The drawing under review shows one solid part. Ordinate dimensions are in mm from its lowest x, y, z. Round coordinates to 2 decimals unless told otherwise and drop trailing zeros. Order: outer loops, then holes, each group sorted by start corner. A loop starts at its lowest first (then second) coordinate and runs counter-clockwise, first axis right, second up. Notation, with made-up numbers: M 43.5,-36.5 L 82.5,-36.5 A13 ccw 82.5,-27.5 Z; hole C 20.5,23 d7. An arc over 180 degrees is marked long. Use a Markdown table: item, result.
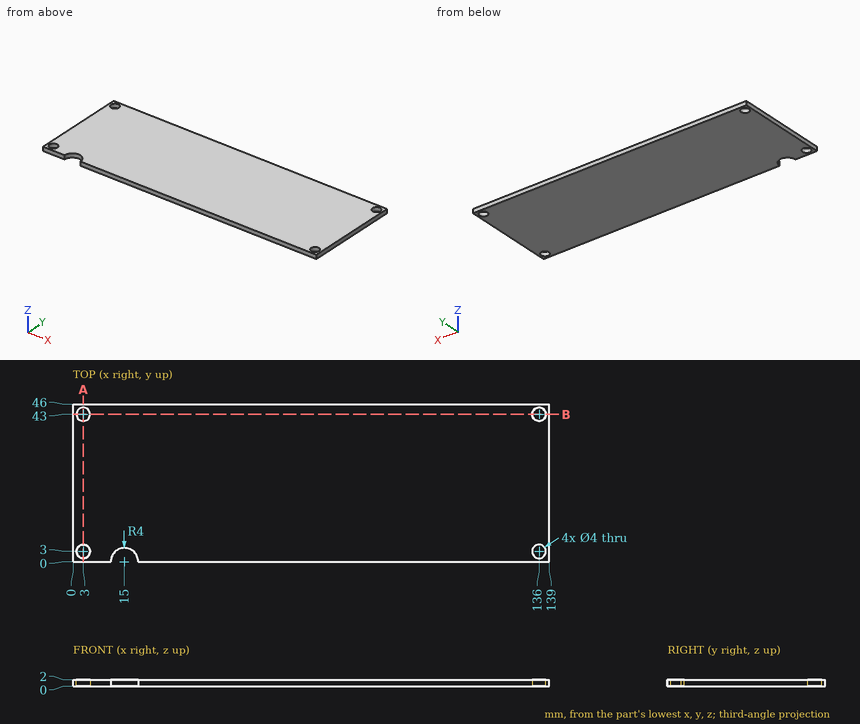
Q1. Add section A-A (x = 3). Write out the cut boundary in (y, z).
Determined:
| item | result |
|---|---|
| outline | M 0,0 L 1,0 L 1,2 L 0,2 Z; M 5,0 L 41,0 L 41,2 L 5,2 Z; M 45,0 L 46,0 L 46,2 L 45,2 Z |
Q2. Wall thickness on line 1 along Y through (x, z) = (136, 1.15); line 2 along X through (y, z) = (3, 0.6); line 3 along X through (y, z) = (42.5, 1.5): over which ranges is each line inside the solid? List them lowest first. Write a range as [from, to].
Determined:
| item | result |
|---|---|
| line 1 | y = [0, 1], [5, 41], [45, 46] |
| line 2 | x = [0, 1], [5, 12.35], [17.65, 134], [138, 139] |
| line 3 | x = [0, 1.06], [4.94, 134.06], [137.94, 139] |
Q3. Add section B-B (y = 43). Write out the cut boundary in (x, z).
Determined:
| item | result |
|---|---|
| outline | M 0,0 L 1,0 L 1,2 L 0,2 Z; M 5,0 L 134,0 L 134,2 L 5,2 Z; M 138,0 L 139,0 L 139,2 L 138,2 Z |
